Geometry: see drawing. Coordinates: mm, zero at the bounding-box minimum. Round coordinates to 2 decimals unless told otherwise and drop trailing zeros. Loops run counter-clockwise (first coordinate to the right, second up) from the corner with the lowest first, then second, coordinate; pieces in that order, holes last. Notation, with made-up numbers: M 11,3 L 53,3 A16 cw 53,20 Z; hole C -18,36.5 d2. An arc over 180 degrees is marked long. Answer as a JSON object with one key per item and string values.
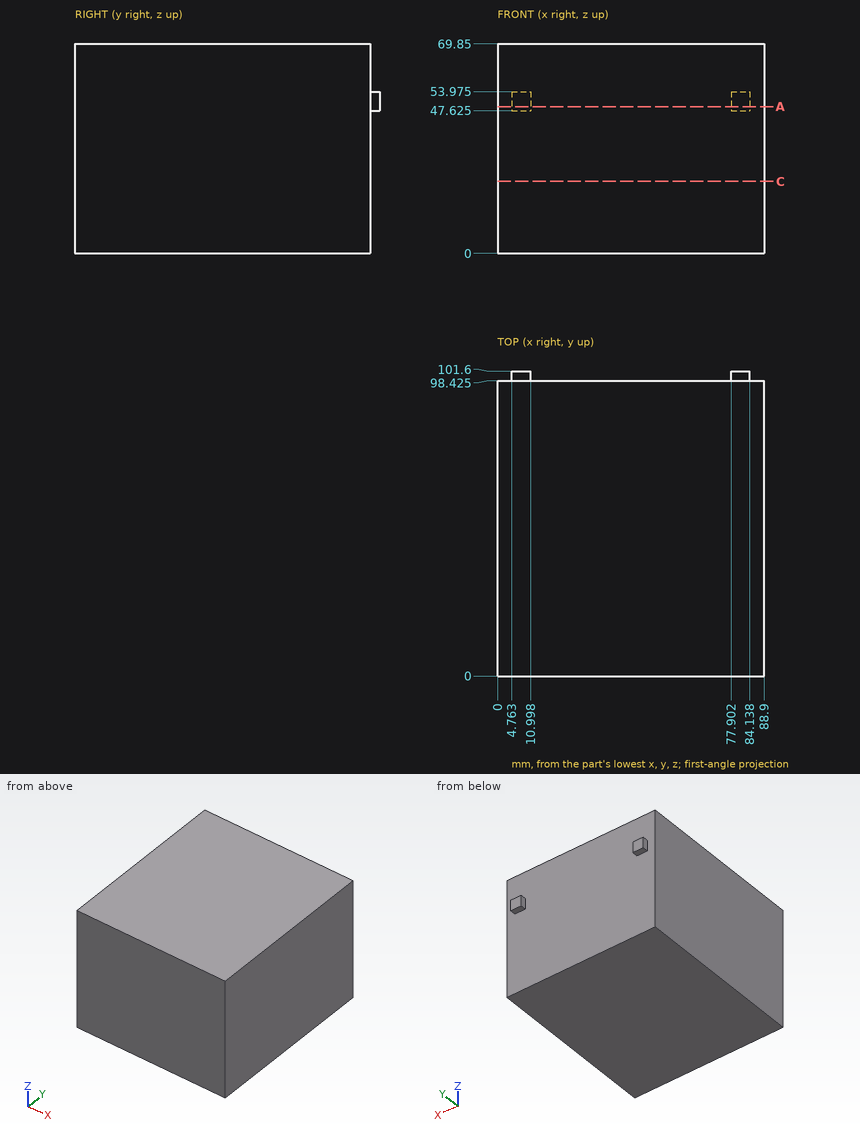
1) Section query C-C (z = 24). Return the cut outline in (x, y) (1 decimal).
Results:
{"outline": "M 0,0 L 88.9,0 L 88.9,98.4 L 0,98.4 Z"}
2) Pin query (flat end, axial travel): P1, Ø10, axis at x = 72, z = 50, coming from the +Y side (1 decimal); P2, Ø3.5, axis at x = 82.5, y = 100.5, coming from the -Z side (1 decimal); P3, Ø2.5, axis at y = 100, z = 52, coming from the -X side. Return the tip coordinate at first contact, or that it passes through.
Results:
{"P1": "y = 98.4", "P2": "z = 47.6", "P3": "x = 4.76"}
3) Ray query, line 1 (Y direction, x = 44, z = 58) (1 decimal). Return the intervals inside material, ascending.
Results:
{"line 1": "0 to 98.4"}
4) Section query A-A (z = 49). Return the cut outline in (x, y) (1 decimal).
Results:
{"outline": "M 0,0 L 88.9,0 L 88.9,98.4 L 84.1,98.4 L 84.1,101.6 L 77.9,101.6 L 77.9,98.4 L 11,98.4 L 11,101.6 L 4.8,101.6 L 4.8,98.4 L 0,98.4 Z"}
